Input: dimensioned drawing with shaded views. Units: mm. Origin: part minimum x, y, z. Coordinates: 2 decimals unless noted, no trailing zeros. Order: outer loops, then holes, each group sorted by start corner. A loop starts at its lowest first (then second) coordinate and runs counter-clockwise, first axis right, second up. Notation, with made-up numbers: (-15.5, 17) -> (2.5, 17) arc R23 cw to (2.5, 53) -> close; hole circle Ø5 at (-16, -3.75). An arc over 180 degrees is marked (long way). Answer in a Markdown table with one row per item. Add a question column.
1) Section query B-B on y = 10. Return the cut outline in (x, z), then the cut area to 3 significant figures.
2) Section query D-D on z = 19. Return the cut outline in (x, y), then the cut area to 3 significant figures.
3) Contact query for flat-ended pins moving along their axis: P1, Ø2, axis at x = 2.5, z = 30.5, coming from the -Y side; P2, Ø12, axis at x = 5.5, z = 35.5, coming from the +Y side; P3, Ø5, axis at x = 15, z = 12, coming from the +Y side. Output: stop coordinate, or through.
4) Ray query, line 1 (Z direction, x = 19, y = 9); line 2 (Z direction, x = 10.5, y = 15.25); line 3 (Y direction, x = 9, z = 43). Return the intervals inside material, ascending. Write a range as from..to.
5) Section query C-C on z = 52. Return the cut outline in (x, y).
6) Section query A-A on x = 10. Return the cut outline in (y, z).
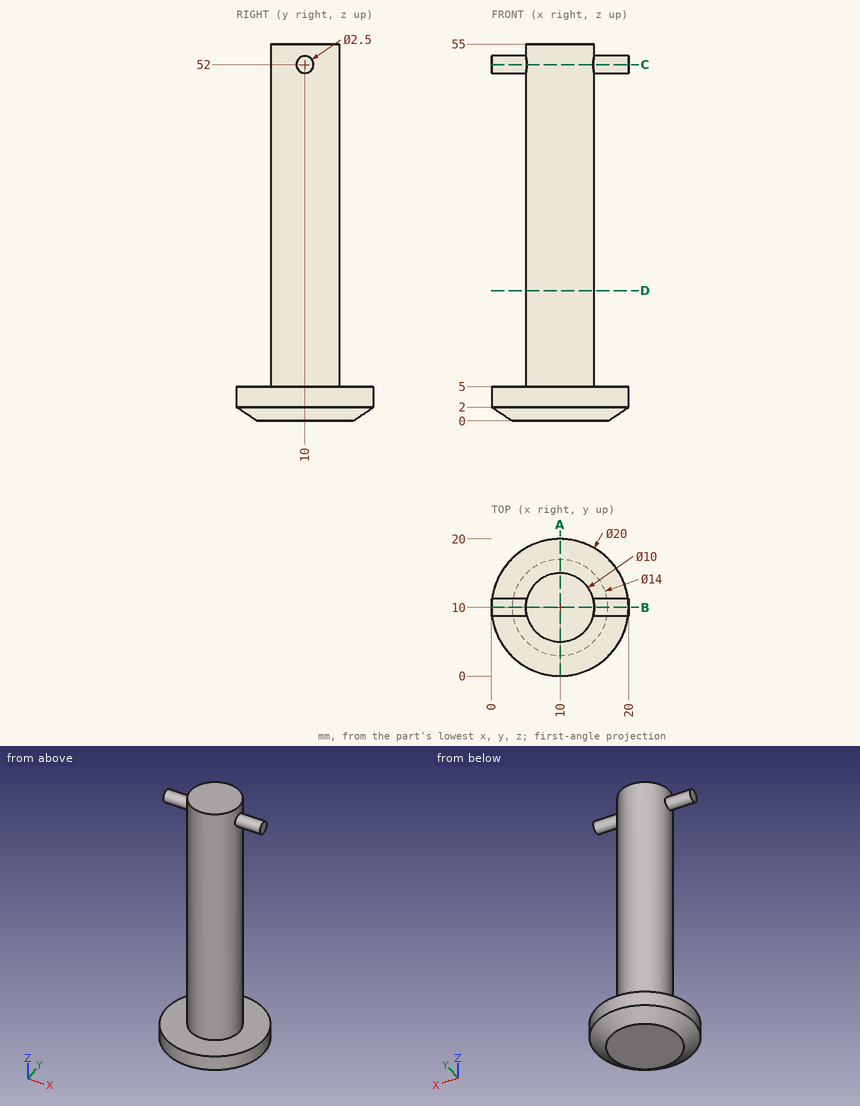
Result:
| question | item | result |
|---|---|---|
| 1 | outline | (0, 2) -> (3, 0) -> (17, 0) -> (20, 2) -> (20, 5) -> (15, 5) -> (15, 50.75) -> (20, 50.75) -> (20, 53.25) -> (15, 53.25) -> (15, 55) -> (5, 55) -> (5, 53.25) -> (0, 53.25) -> (0, 50.75) -> (5, 50.75) -> (5, 5) -> (0, 5) -> close |
| 1 | area | 619 mm2 |
| 2 | outline | circle Ø10 at (10, 10) |
| 2 | area | 78.5 mm2 |
| 3 | P1 | through |
| 3 | P2 | y = 15 |
| 3 | P3 | y = 14.33 |
| 4 | line 1 | 1.37..5, 51.25..52.75 |
| 4 | line 2 | 0..5 |
| 4 | line 3 | 5.1..14.9 |
| 5 | outline | (0, 8.75) -> (5.16, 8.75) arc R5 ccw to (14.84, 8.75) -> (20, 8.75) -> (20, 11.25) -> (14.84, 11.25) arc R5 ccw to (5.16, 11.25) -> (0, 11.25) -> close |
| 6 | outline | (0, 2) -> (3, 0) -> (17, 0) -> (20, 2) -> (20, 5) -> (15, 5) -> (15, 55) -> (5, 55) -> (5, 5) -> (0, 5) -> close |
